```python
from build123d import *

# Parameters (mm, degrees)
F0_W     = 96.331384033
F0_H     = 66.804073751
F1_DEPTH = 50.8
F2_W     = 86.2758494914
F2_H     = 58.5615355521
F3_DEPTH = 45.72
F4_W     = 42.655935511
F4_H     = 20.9858628541
F5_DEPTH = 25.4
F6_W     = 46.9938255847
F6_H     = 20.7962493032
F7_DEPTH = 25.4
F8_R     = 7.7718220909
F9_DEPTH = 127


with BuildPart() as f1:
    # F0 (on Top) → F1 (new body)
    with BuildSketch(Plane.XY):
        with Locations((-1.048495993, 11.8953883648)):
            Rectangle(F0_W, F0_H)
    extrude(amount=F1_DEPTH)

    # F2 (on face) → F3 (cut)
    with BuildSketch(Plane.XY.offset(50.8)):
        with Locations((-0.8434783667, 11.5677108988)):
            Rectangle(F2_W, F2_H)
    extrude(amount=-F3_DEPTH, mode=Mode.SUBTRACT)

    # F4 (on face) → F5 (cut)
    with BuildSketch(Plane.XZ.offset(21.5066485107)):
        with Locations((0.7229829207, 40.3070685729)):
            Rectangle(F4_W, F4_H)
    extrude(amount=-F5_DEPTH, mode=Mode.SUBTRACT)

    # F6 (on face) → F7 (cut)
    with BuildSketch(Plane(origin=(0, 45.2974252403, 0), x_dir=(-1, 0, 0), z_dir=(0, 1, 0))):
        with Locations((4.096897319, 40.4018753484)):
            Rectangle(F6_W, F6_H)
    extrude(amount=-F7_DEPTH, mode=Mode.SUBTRACT)

    # F8 (on face) → F9 (cut)
    with BuildSketch(Plane.YZ.offset(47.1171960235)):
        with Locations((11.2062208354, 26.8708299845)):
            Circle(F8_R)
    extrude(amount=-F9_DEPTH, mode=Mode.SUBTRACT)


solid = f1.part
```
Input: part model. Units: mm. Frame: model coordinates. A direction names the side the tool comes from. Give positions to 0.01 mm unless a question says otherwise; leave off trailing zeros. Order: outer loops, then holes, each group sorted by start corner. A loop starts at its lowest first (then second) coordinate and runs counter-clockwise, first axis right, second up. Notation, with made-up numbers: M 85.5,77 L 90.5,77 A14 ccw 90.5,104 Z; hole C -11,12.25 d6. An arc over 180 degrees is marked long. Return JSON: item names as keys, results as strings.
1) Section query D-D on x = 12. Output: boundary loops of the cut face in (y, z).
Taken from the geometry:
{"outline": "M -21.51,0 L 45.3,0 L 45.3,30 L 40.85,30 L 40.85,5.08 L -17.71,5.08 L -17.71,29.81 L -21.51,29.81 Z"}
2) Section query C-C on z = 17. Output: boundary loops of the cut face in (x, y), and give its area (3 significant figures).
Taken from the geometry:
{"outline": "M -49.21,-21.51 L 47.12,-21.51 L 47.12,45.3 L -49.21,45.3 Z; hole M -43.98,-17.71 L 42.29,-17.71 L 42.29,40.85 L -43.98,40.85 Z", "area": "1,380 mm2"}
3) Section query B-B on y = 9. Output: boundary loops of the cut face in (x, z).
Taken from the geometry:
{"outline": "M -49.21,0 L 47.12,0 L 47.12,19.42 L 42.29,19.42 L 42.29,5.08 L -43.98,5.08 L -43.98,19.42 L -49.21,19.42 Z; M -49.21,34.32 L -43.98,34.32 L -43.98,50.8 L -49.21,50.8 Z; M 42.29,34.32 L 47.12,34.32 L 47.12,50.8 L 42.29,50.8 Z"}
4) Access query for faces 1 (the face through (19.4, 43, 40)), 2 (the face through (42.294, 5, 33)), 3 (the face through (0, -20, 29.814)). Directions: +Z, -Z, +X, -X, +Y, -Y. A direction counts if a zero-diameter tool reaches every point of the face in a straight line with its end or side. Return the directions, or none.
Taken from the geometry:
{"face 1": "+Z, +Y, -Y", "face 2": "+Z", "face 3": "+Z, -Y"}
5) Section query A-A on z = 46. Output: boundary loops of the cut face in (x, y).
Taken from the geometry:
{"outline": "M -49.21,-21.51 L -20.6,-21.51 L -20.6,-17.71 L -43.98,-17.71 L -43.98,40.85 L -27.59,40.85 L -27.59,45.3 L -49.21,45.3 Z; M 19.4,40.85 L 42.29,40.85 L 42.29,-17.71 L 22.05,-17.71 L 22.05,-21.51 L 47.12,-21.51 L 47.12,45.3 L 19.4,45.3 Z"}
6) Contact query for flat-ended pins moving along their axis: pin 1 (8 mm diameter, centred on x = -14, y = 1, fed in from -Z); pin 2 (3.5 mm diameter, centred on x = -3, y = 42, fed in from +Z); pin 3 (12.5 mm diameter, centred on y = 11.21, z = 26.87, fed in from -X); pin 4 (4 mm diameter, centred on x = 18, z = 37, fed in from -Y). Output: stop coordinate, or through.
Taken from the geometry:
{"pin 1": "stops at z = 0", "pin 2": "stops at z = 30", "pin 3": "passes through", "pin 4": "stops at y = 40.85"}
7) Line query: L1, parallel to X at y = 33.5, z = 30.5; L2, parallel to Y at x = 4.5, z = 13; L3, parallel to X at y = 41, z = 40.5. Output: solid intervals per line, ascending. Write a range as [from, to].
Taken from the geometry:
{"L1": "x = [-49.21, -43.98], [42.29, 47.12]", "L2": "y = [-21.51, -17.71], [40.85, 45.3]", "L3": "x = [-49.21, -27.59], [19.4, 47.12]"}
8) Mould query, pull axis X, two halves, no side actions, for faces 4 (the face through (-2, -21.507, 19)), 5 (the face through (-49.214, 19, 25)), 6 (the face through (-1, 12, 5.08)), 7 (the face through (47.117, 19, 25)). Classes: released by +X, released by -X, zero draft, split by the parting line, or undercut.
Taken from the geometry:
{"face 4": "zero draft", "face 5": "released by -X", "face 6": "undercut", "face 7": "released by +X"}
